from build123d import *

# Parameters (mm, degrees)
SKETCH1_R                       = 2.3495
SKETCH1_R_2                     = 1.9812
EXTRUDE1_DEPTH                  = 1.190625
SKETCH6_R                       = 1.5875
SKETCH6_R_2                     = 0.79375
EXTRUDE3_DEPTH                  = 0.6096
SKETCH7_R                       = 3
SKETCH7_R_2                     = 1.9812
EXTRUDE4_DEPTH                  = 4.445
SKETCH16_R                      = 3.937
SKETCH16_R_2                    = 3
EXTRUDE11_DEPTH                 = 1.905
CUT_EXTRUDE1_REACH              = 24.444
SKETCH11_R                      = 7.874
SKETCH11_R_2                    = 6.604
EXTRUDE6_DEPTH                  = 4.572
SKETCH10_W                      = 37.211
SKETCH10_H                      = 18.161
EXTRUDE5_DEPTH                  = 22.225
SKETCH13_W                      = 1.143
SKETCH13_H                      = 3.048
EXTRUDE8_DEPTH                  = 10.795
EXTRUDE9_START                  = -1.952625
SKETCH14_R                      = 0.79375
EXTRUDE9_DEPTH                  = 22.987
SKETCH23_R                      = 0.79375
CUT_EXTRUDE2_DEPTH              = 1.190625
CUT_EXTRUDE3_REACH              = 36.655
MIRROR2_START                   = -1.952625
MIRROR2_COPY_1_SKETCH_R         = 0.79375
MIRROR2_COPY_1_DEPTH            = 22.987
SKETCH18_W                      = 36.195
SKETCH18_H                      = 17.145
EXTRUDE12_DEPTH                 = 0.762
SKETCH19_R                      = 2.54
EXTRUDE13_DEPTH                 = 1.905
EXTRUDE14_DEPTH                 = 5.588
F_1_64_TAPPED_HOLE1_D           = 1.5113
F_1_64_TAPPED_HOLE1_DEPTH       = 5.588
F_1_64_TAPPED_HOLE1_CBORE_D     = 1.8542
F_1_64_TAPPED_HOLE1_CBORE_DEPTH = 3.7084


with BuildPart() as part:
    # Sketch1 → Extrude1 (new body)
    with BuildSketch(Plane(origin=(0, 0, 0), x_dir=(1, 0, 0), z_dir=(0, 1, 0))):
        with BuildLine():
            Line((-18.6055, 9.8425), (18.6055, 9.8425))
            ThreePointArc((18.6055, 9.8425), (19.144315367, 9.619315367), (19.3675, 9.0805))
            Line((19.3675, 9.0805), (19.3675, -9.0805))
            ThreePointArc((19.3675, -9.0805), (19.144315367, -9.619315367), (18.6055, -9.8425))
            Line((18.6055, -9.8425), (-18.6055, -9.8425))
            ThreePointArc((-18.6055, -9.8425), (-19.144315367, -9.619315367), (-19.3675, -9.0805))
            Line((-19.3675, -9.0805), (-19.3675, 9.0805))
            ThreePointArc((-19.3675, 9.0805), (-19.144315367, 9.619315367), (-18.6055, 9.8425))
        make_face()
        with Locations(Location((-11.049, 0, 0), (0, 0, 90))):
            Circle(SKETCH1_R, mode=Mode.SUBTRACT)
        with Locations(Location((9.525, 0, 0), (0, 0, 90))):
            Circle(SKETCH1_R_2, mode=Mode.SUBTRACT)
    extrude(amount=EXTRUDE1_DEPTH)

    # Sketch6 → Extrude3 (add)
    with BuildSketch(Plane(origin=(0, 1.190625, 0), x_dir=(-1, 0, 0), z_dir=(0, 1, 0))):
        with Locations(Location((1.8415, 0, 0), (0, 0, 270))):
            Circle(SKETCH6_R)
        with Locations(Location((1.8415, 0, 0), (0, 0, 90))):
            Circle(SKETCH6_R_2, mode=Mode.SUBTRACT)
    extrude(amount=EXTRUDE3_DEPTH)

    # Sketch7 → Extrude4 (add)
    with BuildSketch(Plane(origin=(0, 1.190625, 0), x_dir=(-1, 0, 0), z_dir=(0, 1, 0))):
        with Locations(Location((-9.525, 0, 0), (0, 0, 270))):
            Circle(SKETCH7_R)
        with Locations(Location((-9.525, 0, 0), (0, 0, 270))):
            Circle(SKETCH7_R_2, mode=Mode.SUBTRACT)
    extrude(amount=EXTRUDE4_DEPTH)

    # Sketch16 → Extrude11 (add)
    with BuildSketch(Plane(origin=(0, 1.190625, 0), x_dir=(-1, 0, 0), z_dir=(0, 1, 0))):
        with Locations(Location((-9.525, 0, 0), (0, 0, 270))):
            Circle(SKETCH16_R)
        with Locations(Location((-9.525, 0, 0), (0, 0, 90))):
            Circle(SKETCH16_R_2, mode=Mode.SUBTRACT)
    extrude(amount=EXTRUDE11_DEPTH)

    # Cut-Extrude1: up to this face of the body (flat: up to its plane)
    cut_extrude1_end = Plane(part.part.faces().sort_by_distance((0, 1.190625, -9.408000351))[0])
    # Sketch17 → Cut-Extrude1 (cut, up to the picked face)
    with BuildSketch(Plane(origin=(0, 5.635625, 0), x_dir=(-1, 0, 0), z_dir=(0, 1, 0)), mode=Mode.PRIVATE) as cut_extrude1_sk1:
        with BuildLine():
            ThreePointArc((-6.516949302, 2.54), (-6.894361419, 0), (-6.516949302, -2.54))
            ThreePointArc((-6.516949302, -2.54), (-5.588, 0), (-6.516949302, 2.54))
        make_face()
    cut_extrude1_tool1 = split(extrude(cut_extrude1_sk1.sketch, amount=-CUT_EXTRUDE1_REACH, mode=Mode.PRIVATE), bisect_by=cut_extrude1_end, keep=Keep.BOTH, mode=Mode.PRIVATE)
    add(cut_extrude1_tool1.solids().sort_by(Axis((6.291228, 5.635625, 0), (0, -1, 0)))[0], mode=Mode.SUBTRACT)

    # Sketch11 → Extrude6 (add)
    with BuildSketch(Plane.XZ):
        with Locations(Location((9.525, 0, 0), (0, 0, 270))):
            Circle(SKETCH11_R)
        with Locations(Location((9.525, 0, 0), (0, 0, 270))):
            Circle(SKETCH11_R_2, mode=Mode.SUBTRACT)
    extrude(amount=EXTRUDE6_DEPTH)

    # Sketch10 → Extrude5 (add)
    with BuildSketch(Plane.XZ.offset(-1.190625)):
        with BuildLine():
            Line((-19.3675, 9.0805), (-19.3675, -9.0805))
            ThreePointArc((-19.3675, -9.0805), (-19.144315367, -9.619315367), (-18.6055, -9.8425))
            Line((-18.6055, -9.8425), (18.6055, -9.8425))
            ThreePointArc((18.6055, -9.8425), (19.144315367, -9.619315367), (19.3675, -9.0805))
            Line((19.3675, -9.0805), (19.3675, 9.0805))
            ThreePointArc((19.3675, 9.0805), (19.144315367, 9.619315367), (18.6055, 9.8425))
            Line((18.6055, 9.8425), (-18.6055, 9.8425))
            ThreePointArc((-18.6055, 9.8425), (-19.144315367, 9.619315367), (-19.3675, 9.0805))
        make_face()
        Rectangle(SKETCH10_W, SKETCH10_H, mode=Mode.SUBTRACT)
    extrude(amount=EXTRUDE5_DEPTH)

    # Sketch13 → Extrude8 (add)
    with BuildSketch(Plane.XZ):
        with BuildLine():
            Line((-5.9055, 6.0325), (-5.9055, 9.0805))
            Line((-5.9055, 9.0805), (-4.7625, 9.0805))
            Line((-4.7625, 9.0805), (-4.7625, 6.713831938))
            ThreePointArc((-4.7625, 6.713831938), (-1.851412189, 0), (-4.7625, -6.713831938))
            Line((-4.7625, -6.713831938), (-4.7625, -9.0805))
            Line((-4.7625, -9.0805), (-5.9055, -9.0805))
            Line((-5.9055, -9.0805), (-5.9055, -6.0325))
            ThreePointArc((-5.9055, -6.0325), (-3.121412189, 0), (-5.9055, 6.0325))
        make_face()
        with Locations((-8.382, 7.5565)):
            Rectangle(SKETCH13_W, SKETCH13_H)
        with Locations((-13.335, 7.5565)):
            Rectangle(SKETCH13_W, SKETCH13_H)
        with Locations((-13.335, -7.5565)):
            Rectangle(SKETCH13_W, SKETCH13_H)
        with Locations((-8.382, -7.5565)):
            Rectangle(SKETCH13_W, SKETCH13_H)
    extrude(amount=EXTRUDE8_DEPTH)

    # Sketch14 → Extrude9 (add)
    with BuildSketch(Plane.XZ.offset(EXTRUDE9_START)):
        with BuildLine():
            Line((-18.6055, -9.0805), (-18.6055, -6.911913297))
            ThreePointArc((-18.6055, -6.911913297), (-16.235418625, -6.710418625), (-16.436913297, -9.0805))
            Line((-16.436913297, -9.0805), (-18.6055, -9.0805))
        make_face()
        with Locations(Location((-17.3355, -7.8105, 0), (0, 0, 270))):
            Circle(SKETCH14_R, mode=Mode.SUBTRACT)
    extrude9 = extrude(amount=EXTRUDE9_DEPTH)

    # Sketch23 → Cut-Extrude2 (cut)
    with BuildSketch(Plane(origin=(0, 1.190625, 0), x_dir=(-1, 0, 0), z_dir=(0, 1, 0))):
        with Locations(Location((17.3355, -7.8105, 0), (0, 0, 270))):
            Circle(SKETCH23_R)
    extrude(amount=-CUT_EXTRUDE2_DEPTH, mode=Mode.SUBTRACT)

    # Sketch9 → Revolve1 (revolve)
    with BuildSketch(Plane.XY, mode=Mode.PRIVATE) as revolve1_sk:
        Polygon((-12.954, 5.965825), (-12.954, 6.550025), (-11.84275, 6.550025), (-11.84275, 5.965825), (-11.049, 5.965825), (-11.049, 4.645025), (-13.3985, 4.645025), (-13.3985, 1.190625), (-15.1765, 1.190625), (-15.1765, 1.952625), (-14.6685, 1.952625), (-14.6685, 5.965825), align=None)
    revolve(revolve1_sk.sketch.rotate(Axis((-11.049, 0, 0), (0, 1, 0)), 270), axis=Axis((-11.049, 0, 0), (0, 1, 0)))

    # Cut-Extrude3: up to this face of the body (flat: up to its plane)
    cut_extrude3_end = Plane(part.part.faces().sort_by_distance((-1.8415, 1.190625, 0))[0])
    # Sketch24 → Cut-Extrude3 (cut, up to the picked face)
    with BuildSketch(Plane(origin=(0, 5.965825, 0), x_dir=(-1, 0, 0), z_dir=(0, 1, 0)), mode=Mode.PRIVATE) as cut_extrude3_sk1:
        with BuildLine():
            Line((10.316307692, 1.758461538), (9.4615, 3.81))
            ThreePointArc((9.4615, 3.81), (6.9215, 0), (9.4615, -3.81))
            Line((9.4615, -3.81), (10.316307692, -1.758461538))
            ThreePointArc((10.316307692, -1.758461538), (9.144, 0), (10.316307692, 1.758461538))
        make_face()
    cut_extrude3_tool1 = split(extrude(cut_extrude3_sk1.sketch, amount=-CUT_EXTRUDE3_REACH, mode=Mode.PRIVATE), bisect_by=cut_extrude3_end, keep=Keep.BOTH, mode=Mode.PRIVATE)
    add(cut_extrude3_tool1.solids().sort_by(Axis((-8.574349, 5.965825, 0), (0, -1, 0)))[0], mode=Mode.SUBTRACT)

    # Mirror1: Extrude9 across plane
    add(extrude9.mirror(Plane(origin=(0, 0, 0), x_dir=(0, 0, 1), z_dir=(1, 0, 0))))

    # Mirror2: Extrude9 across plane
    add(extrude9.mirror(Plane.XY))

    # Mirror2 copy 1 sketch → Mirror2 copy 1 (add)
    with BuildSketch(Plane(origin=(0, 0, 0), x_dir=(-1, 0, 0), z_dir=(0, -1, 0)).offset(MIRROR2_START)):
        with BuildLine():
            Line((-18.6055, -9.0805), (-18.6055, -6.911913297))
            ThreePointArc((-18.6055, -6.911913297), (-16.235418625, -6.710418625), (-16.436913297, -9.0805))
            Line((-16.436913297, -9.0805), (-18.6055, -9.0805))
        make_face()
        with Locations(Location((-17.3355, -7.8105, 0), (0, 0, 270))):
            Circle(MIRROR2_COPY_1_SKETCH_R, mode=Mode.SUBTRACT)
    extrude(amount=MIRROR2_COPY_1_DEPTH)

    # Sketch18 → Extrude12 (add)
    with BuildSketch(Plane(origin=(0, 1.952625, 0), x_dir=(-1, 0, 0), z_dir=(0, 1, 0))):
        with BuildLine():
            Line((18.6055, 9.2075), (-18.6055, 9.2075))
            ThreePointArc((-18.6055, 9.2075), (-18.695302561, 9.170302561), (-18.7325, 9.0805))
            Line((-18.7325, 9.0805), (-18.7325, -9.0805))
            ThreePointArc((-18.7325, -9.0805), (-18.695302561, -9.170302561), (-18.6055, -9.2075))
            Line((-18.6055, -9.2075), (18.6055, -9.2075))
            ThreePointArc((18.6055, -9.2075), (18.695302561, -9.170302561), (18.7325, -9.0805))
            Line((18.7325, -9.0805), (18.7325, 9.0805))
            ThreePointArc((18.7325, 9.0805), (18.695302561, 9.170302561), (18.6055, 9.2075))
        make_face()
        Rectangle(SKETCH18_W, SKETCH18_H, mode=Mode.SUBTRACT)
    extrude(amount=-EXTRUDE12_DEPTH)

    # Sketch19 → Extrude13 (add)
    with BuildSketch(Plane.XZ):
        with BuildLine():
            Line((11.557, -3.222898695), (11.557, -6.283612973))
            ThreePointArc((11.557, -6.283612973), (11.178939296, -6.393535861), (10.795, -6.480734218))
            Line((10.795, -6.480734218), (10.795, -3.592102448))
            ThreePointArc((10.795, -3.592102448), (9.525, -3.81), (8.255, -3.592102448))
            Line((8.255, -3.592102448), (8.255, -6.480734218))
            ThreePointArc((8.255, -6.480734218), (7.871060704, -6.393535861), (7.493, -6.283612973))
            Line((7.493, -6.283612973), (7.493, -3.222898695))
            ThreePointArc((7.493, -3.222898695), (9.525, 3.81), (11.557, -3.222898695))
        make_face()
        with Locations(Location((9.525, 0, 0), (0, 0, 90))):
            Circle(SKETCH19_R, mode=Mode.SUBTRACT)
    extrude(amount=EXTRUDE13_DEPTH)

    # Sketch20 → Extrude14 (add)
    with BuildSketch(Plane.XZ):
        with BuildLine():
            ThreePointArc((4.320531036, -4.065257532), (3.147336001, -7.413112903), (6.282470752, -5.753157401))
            ThreePointArc((6.282470752, -5.753157401), (5.218006131, -5.006258065), (4.320531036, -4.065257532))
        make_face()
    extrude(amount=EXTRUDE14_DEPTH)

    # 1-64 Tapped Hole1
    with Locations(Plane(origin=(4.389738079, -5.588, -5.969), x_dir=(0, 0, -1), z_dir=(0, -1, 0))):
        with Locations((0, 0)):
            CounterBoreHole(F_1_64_TAPPED_HOLE1_D / 2, F_1_64_TAPPED_HOLE1_CBORE_D / 2, F_1_64_TAPPED_HOLE1_CBORE_DEPTH, depth=F_1_64_TAPPED_HOLE1_DEPTH)


solid = part.part
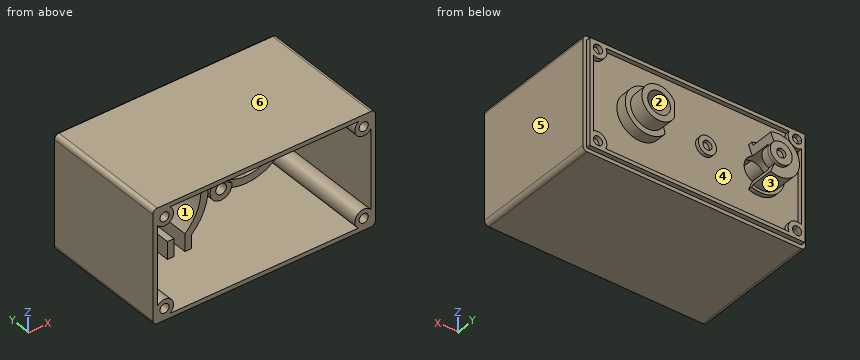
Verification items for the finished model (mm, model axes). Face numbers are marked on the shaded views. A direction names the side the tool comes from. Coordinates: 2 decimals unless noted, no trailing zeros. Order: outer loops, then holes, each group sorted by start corner. A loop starts at its lowest first (then second) coordinate and runs counter-clockwise, first axis right, second up.
Item 1: Section check B-B, the plane z = 0. Give the number of separate pieces and of enclosed holes in the cut face, then the cut area to 3 significant figures.
Filled in:
separate pieces: 3
enclosed holes: 0
area: 123 mm2
Item 2: Material ranges on L1, parallel to Z at x = 12, y = -17.5; L2, parallel to X at y = -3, z = 3.5; L3, parallel to X at y = -9.25, z = 2.5, recorded low to high.
Filled in:
L1: z = -9.84 to -9.08, 9.08 to 9.84
L2: x = -19.37 to -18.61, -3.94 to -2.54, 2.47 to 3.92, 15.13 to 16.58, 18.61 to 19.37
L3: x = -19.37 to -18.61, -3.53 to -2.2, 18.61 to 19.37
Item 3: Depth check by flat-ended pin: pin 1 (2 mm diameter, centred on x = 17.34, z = 7.81, fed in from +Y); pin 2 (2 mm diameter, centred on x = 4, z = 5.5, fed in from -Y); pin 3 (4.5 mm diameter, centred on x = -10.5, z = 2, fed in from -Y). Enter the tip coordinate at first touch or a pass-through.
Filled in:
pin 1: stops at y = 1.95
pin 2: stops at y = -4.57
pin 3: stops at y = 0
Item 4: Release check for a two-part mould opening along Z. For the marked faces 3, 4, 5 and 6 record: +Z half, -Z half, draft (parallel to the pull), parting line (faces both ways), or undercut.
Filled in:
face 3: parting line
face 4: undercut
face 5: draft
face 6: +Z half
Item 5: Section check A-A, the plane y = -16.75. Enter the section's corners in (x, z), then the cut area to 3 significant figures.
Filled in:
outline: (-19.37, -9.08) arc R0.76 ccw to (-18.61, -9.84) - (18.61, -9.84) arc R0.76 ccw to (19.37, -9.08) - (19.37, 9.08) arc R0.76 ccw to (18.61, 9.84) - (-18.61, 9.84) arc R0.76 ccw to (-19.37, 9.08) - close; hole (-18.61, -6.91) arc R1.56 cw (long way) to (-16.44, -9.08) - (16.44, -9.08) arc R1.56 cw (long way) to (18.61, -6.91) - (18.61, 6.91) arc R1.56 cw (long way) to (16.44, 9.08) - (-16.44, 9.08) arc R1.56 cw (long way) to (-18.61, 6.91) - close; hole circle Ø1.59 at (-17.34, -7.81); hole circle Ø1.59 at (-17.34, 7.81); hole circle Ø1.59 at (17.34, -7.81); hole circle Ø1.59 at (17.34, 7.81)
area: 106 mm2
Item 6: Section check C-C, the plane x = 1. Enter the section's corners in (y, z), then the cut area to 3 significant figures.
Filled in:
outline: (-21.03, -9.84) - (1.19, -9.84) - (1.19, -9.21) - (1.95, -9.21) - (1.95, -8.57) - (1.19, -8.57) - (1.19, 8.57) - (1.95, 8.57) - (1.95, 9.21) - (1.19, 9.21) - (1.19, 9.84) - (-21.03, 9.84) - (-21.03, 9.08) - (0, 9.08) - (0, -9.08) - (-21.03, -9.08) - close
area: 56.5 mm2
Item 7: Access from +Z, -Z, +X, -X, +Y, -Y to the whole of each face (thin tool, end or side, straight path). Record for the marked faces 1 and 2.
Filled in:
face 1: -Y
face 2: +Y, -Y
